```python
from build123d import *

# Parameters (mm, degrees)
SKETCH1_R            = 45.974
SKETCH1_R_2          = 27.4955
SKETCH1_R_3          = 6.5
BOSS_EXTRUDE1_DEPTH  = 6.04774
M8_CLEARANCE_HOLE1_D = 9
CIRPATTERN1_COUNT    = 18
CUT_EXTRUDE1_DEPTH   = 66.297722097
FILLET1_R            = 1.5875
FILLET1_OF_MIRROR1_R = 1.5875


with BuildPart() as part:
    # Sketch1 → Boss-Extrude1 (new body)
    with BuildSketch(Plane(origin=(0, 0, 0), x_dir=(1, 0, 0), z_dir=(0, 1, 0))):
        with Locations(Location((0, 0, 0), (0, 0, 270))):
            Circle(SKETCH1_R)
        with Locations(Location((0, 0, 0), (0, 0, 270))):
            Circle(SKETCH1_R_2, mode=Mode.SUBTRACT)
        with Locations(Location((-13.33878559, -36.648012211, 0), (0, 0, 270))):
            Circle(SKETCH1_R_3, mode=Mode.SUBTRACT)
        with Locations(Location((13.33878559, -36.648012211, 0), (0, 0, 270))):
            Circle(SKETCH1_R_3, mode=Mode.SUBTRACT)
    extrude(amount=BOSS_EXTRUDE1_DEPTH)

    # M8 Clearance Hole1 (through all)
    with Locations(Plane(origin=(0, 6.04774, 0), x_dir=(1, 0, 0), z_dir=(0, 1, 0))):
        with Locations((0, 39)):
            m8_clearance_hole1 = Hole(M8_CLEARANCE_HOLE1_D / 2)

    # CirPattern1: M8 Clearance Hole1 ×18 about axis, 10 skipped
    cirpattern1_axis = Axis((0, 6.04774, 0), (0, -1, 0))
    add([m8_clearance_hole1.rotate(cirpattern1_axis, i * 360 / CIRPATTERN1_COUNT) for i in range(1, CIRPATTERN1_COUNT) if i not in (1, 3, 5, 7, 8, 10, 11, 13, 15, 17)], mode=Mode.SUBTRACT)

    # Sketch6 → Cut-Extrude1 (cut, through all)
    with BuildSketch(Plane(origin=(0, 6.04774, 0), x_dir=(1, 0, 0), z_dir=(0, 1, 0))):
        with BuildLine():
            ThreePointArc((-7.230783555, -38.871143142), (-15.561916521, -42.756014246), (-19.446787625, -34.424881279))
            Line((-19.446787625, -34.424881279), (-21.674084917, -40.544330295))
            ThreePointArc((-21.674084917, -40.544330295), (-15.724034069, -43.201428548), (-9.458080846, -44.990592158))
            Line((-9.458080846, -44.990592158), (-7.230783555, -38.871143142))
        make_face()
    cut_extrude1 = extrude(amount=-CUT_EXTRUDE1_DEPTH, mode=Mode.SUBTRACT)

    # Fillet1
    fillet1_edges = [part.edges().sort_by_distance(p)[0] for p in [
        (-9.458080846, 3.02387, 44.990592158),
        (-21.674084917, 3.02387, 40.544330295),
    ]]
    fillet(fillet1_edges, radius=FILLET1_R)

    # Mirror1: Cut-Extrude1 across plane
    add(cut_extrude1.mirror(Plane(origin=(0, 0, 0), x_dir=(0, 0, 1), z_dir=(1, 0, 0))), mode=Mode.SUBTRACT)

    # Fillet1 of Mirror1
    fillet1_of_mirror1_edges = [part.edges().sort_by_distance(p)[0] for p in [
        (9.458080846, 3.02387, 44.990592158),
        (21.674084917, 3.02387, 40.544330295),
    ]]
    fillet(fillet1_of_mirror1_edges, radius=FILLET1_OF_MIRROR1_R)


solid = part.part
```
Here's how the part is built. I have some questions about the finished solid (model axes, mm). A direction names the side the tool comes from. Give positions to 0.01 mm unless a question says otherwise; leave off trailing zeros. Loops run counter-clockwise (first coordinate to the right, second up) from the corner with the lowest first, then second, coordinate; pieces in that order, holes last. Notation, with made-up numbers: M -7,-21 L 17,-21 A32 ccw 17,14 Z; hole C 34,66 d2. An arc over 180 degrees is marked long. Use one line per item in the form item = value. Start each with the question number.
Q1. Thinking about a two-plate mould opening in Z: for faces 4 (the cylindrical face through (-22.009, 2.982, 39.746)), 5 (the cylindrical face through (28.4, 3, -32.9)), 6 (the cylindrical face through (1.679, 2.982, -45.943)), 7 (the cylindrical face through (-10.98, 2.98, 30.59)), which applies, +Z half, -Z half, draft (parallel to the pull), parting line (faces both ways), or undercut?
Q2. If we section it at B-B (z = 0): Write out the boundary of the cut face in (x, y).
Q3. If we section it at C-C (x = 26): Write out the boundary of the cut face in (y, z).
Q4. If we section it at D-D (z = 32): Write out the boundary of the cut face in (x, y) (3 decimals), then the cut area to 3 significant figures.
Q5. I need wall thicknesses on line 1 along X through (y, z) = (3, -3.5); line 2 along X through (y, z) = (5.5, -7); line 3 along Z through (x, y) = (39, 5). Which ranges of each line are inside material? Lowest first, please.
Q6. If we section it at A-A (x = 0): Write out the boundary of the cut face in (y, z).
Q7. Which directions (+Z, -Z, +X, -X, +Y, -Y) give clear straight access to the entire face, cutting with the end or side of a thin tool? Please do faces 1 (the flat face through (-20, 6.048, -21)), 2 (the flat face through (20.23, 3.07, 36.58)), 3 (the flat face through (8.036, 3.066, 41.083)).
Q8. Will these pins go through, and if not, where does the flat tip stop? pin 1 Ø1 at (y, z) = (1.5, -16) entering from +X; pin 2 Ø8 at (x, z) = (25.07, -29.88) entering from +Y; pin 3 Ø3 at (x, y) = (-4, 2) entering from -Z.
Taken from the geometry:
q1.face_4 = +Z half
q1.face_5 = undercut
q1.face_6 = parting line
q1.face_7 = undercut
q2.outline = M -45.97,0 L -27.5,0 L -27.5,6.05 L -45.97,6.05 Z; M 27.5,0 L 45.97,0 L 45.97,6.05 L 27.5,6.05 Z
q3.outline = M 0,-37.92 L 6.05,-37.92 L 6.05,-34.28 L 0,-34.28 Z; M 0,-25.47 L 6.05,-25.47 L 6.05,-8.94 L 0,-8.94 Z; M 0,8.94 L 6.05,8.94 L 6.05,37.92 L 0,37.92 Z
q4.outline = M -33.009,0 L -17.883,0 L -17.883,6.048 L -33.009,6.048 Z; M -8.795,0 L 8.795,0 L 8.795,6.048 L -8.795,6.048 Z; M 17.883,0 L 33.009,0 L 33.009,6.048 L 17.883,6.048 Z
q4.area = 289 mm^2
q5.line_1 = -45.84 to -41.5, -35.32 to -27.27, 27.27 to 35.32, 41.5 to 45.84
q5.line_2 = -45.44 to -42.9, -33.91 to -26.59, 26.59 to 33.91, 42.9 to 45.44
q5.line_3 = -24.34 to -11.23, -2.31 to 24.34
q6.outline = M 0,-45.97 L 6.05,-45.97 L 6.05,-43.5 L 0,-43.5 Z; M 0,-34.5 L 6.05,-34.5 L 6.05,-27.5 L 0,-27.5 Z; M 0,27.5 L 6.05,27.5 L 6.05,34.5 L 0,34.5 Z; M 0,43.5 L 6.05,43.5 L 6.05,45.97 L 0,45.97 Z
q7.face_1 = +Z, -Z, +X, -X, +Y
q7.face_2 = +Z, +Y, -Y
q7.face_3 = +Y, -Y
q8.pin_1 = 43.28
q8.pin_2 = through
q8.pin_3 = -45.91
